The model under review builds one solid part; all positions refer to its coordinate system, in mm. Face numbers are marked on the shaded views. Coordinates: 2 decimals unless noted, no trailing zeros. Order: outer loops, then holes, each group sorted by start corner. A loop starts at its lowest first (then second) coordinate and runs counter-clockwise, first axis right, second up. Notation, with made-up numbers: (32, 23.25) -> (54, 23.25) arc R23 ccw to (54, 50.25) -> close; hole circle Ø5 at (53.25, -30). An arc over 180 degrees is marked (long way). Put each result on its own line as item: value.
from build123d import *

# Parameters (mm, degrees)
SKETCH1_R             = 100
SKETCH1_R_2           = 40
BOSS_EXTRUDE1_DEPTH   = 5
F_4_0MM_DOWEL_HOLE1_D = 4
SKETCH6_R             = 95
SKETCH6_R_2           = 90
BOSS_EXTRUDE2_DEPTH   = 10
F_4_0MM_DOWEL_HOLE2_D = 4
CUT_EXTRUDE1_DEPTH    = 142.774468788
CIRPATTERN1_DEPTH     = 5
CUT_EXTRUDE2_START    = -10
SKETCH10_R            = 95
SKETCH10_R_2          = 94.5
CUT_EXTRUDE2_DEPTH    = 10
BOSS_EXTRUDE3_DEPTH   = 10


# Read off the part's stored shape, not the designer's step: CirPattern1
with BuildPart() as part:
    # Sketch1 → Boss-Extrude1 (new body)
    with BuildSketch(Plane(origin=(0, 0, 0), x_dir=(1, 0, 0), z_dir=(0, 1, 0))):
        with Locations(Location((0, 0, 0), (0, 0, 270))):
            Circle(SKETCH1_R)
        with Locations(Location((0, 0, 0), (0, 0, 270))):
            Circle(SKETCH1_R_2, mode=Mode.SUBTRACT)
    extrude(amount=BOSS_EXTRUDE1_DEPTH)

    # Ø4.0mm Dowel Hole1 (through all)
    with Locations(Plane(origin=(0, 5, 0), x_dir=(1, 0, 0), z_dir=(0, 1, 0))):
        with Locations((0, 0), (40.5, 40.5), (-40.5, -40.5), (-40.5, 40.5), (40.5, -40.5)):
            Hole(F_4_0MM_DOWEL_HOLE1_D / 2)

    # Sketch6 → Boss-Extrude2 (add)
    with BuildSketch(Plane(origin=(0, 5, 0), x_dir=(1, 0, 0), z_dir=(0, 1, 0))):
        with Locations(Location((0, 0, 0), (0, 0, 270))):
            Circle(SKETCH6_R)
        with Locations(Location((0, 0, 0), (0, 0, 270))):
            Circle(SKETCH6_R_2, mode=Mode.SUBTRACT)
    extrude(amount=BOSS_EXTRUDE2_DEPTH)

    # Ø4.0mm Dowel Hole2 (through all)
    with Locations(Plane(origin=(0, 5, 0), x_dir=(1, 0, 0), z_dir=(0, 1, 0))):
        with Locations((0, 0), (75, 20), (-75, -20), (-75, 20), (75, -20), (20, 75), (-20, -75), (-20, 75), (20, -75), (20, 55), (-20, -55), (-20, 55), (20, -55), (55, -20), (-55, 20), (-55, -20), (55, 20)):
            Hole(F_4_0MM_DOWEL_HOLE2_D / 2)

    # Sketch9 → Cut-Extrude1 (cut, through all)
    with BuildSketch(Plane(origin=(0, 5, 0), x_dir=(1, 0, 0), z_dir=(0, 1, 0))):
        with BuildLine():
            Line((81.567700833, -38.035643557), (59.537983888, -27.763017838))
            ThreePointArc((59.537983888, -27.763017838), (46.451892776, -46.451892776), (27.763017838, -59.537983888))
            Line((27.763017838, -59.537983888), (38.035643557, -81.567700833))
            ThreePointArc((38.035643557, -81.567700833), (63.639610307, -63.639610307), (81.567700833, -38.035643557))
        make_face()
    extrude(amount=-CUT_EXTRUDE1_DEPTH, mode=Mode.SUBTRACT)

    # CirPattern1 outline → CirPattern1 (cut)
    with BuildSketch(Plane(origin=(0, 0, 0), x_dir=(1, 0, 0), z_dir=(0, 1, 0))):
        with BuildLine():
            Line((59.537983888, 27.763017838), (81.567700833, 38.035643557))
            ThreePointArc((81.567700833, 38.035643557), (63.639610307, 63.639610307), (38.035643557, 81.567700833))
            Line((38.035643557, 81.567700833), (27.763017838, 59.537983888))
            ThreePointArc((27.763017838, 59.537983888), (46.451892776, 46.451892776), (59.537983888, 27.763017838))
        make_face()
        with BuildLine():
            ThreePointArc((-81.567700833, -38.035643557), (-63.639610307, -63.639610307), (-38.035643557, -81.567700833))
            Line((-38.035643557, -81.567700833), (-27.763017838, -59.537983888))
            ThreePointArc((-27.763017838, -59.537983888), (-46.451892776, -46.451892776), (-59.537983888, -27.763017838))
            Line((-59.537983888, -27.763017838), (-81.567700833, -38.035643557))
        make_face()
        with BuildLine():
            Line((-27.763017838, 59.537983888), (-38.035643557, 81.567700833))
            ThreePointArc((-38.035643557, 81.567700833), (-63.639610307, 63.639610307), (-81.567700833, 38.035643557))
            Line((-81.567700833, 38.035643557), (-59.537983888, 27.763017838))
            ThreePointArc((-59.537983888, 27.763017838), (-46.451892776, 46.451892776), (-27.763017838, 59.537983888))
        make_face()
    extrude(amount=CIRPATTERN1_DEPTH, mode=Mode.SUBTRACT)

    # Sketch10 → Cut-Extrude2 (cut)
    with BuildSketch(Plane(origin=(0, 15, 0), x_dir=(1, 0, 0), z_dir=(0, 1, 0)).offset(CUT_EXTRUDE2_START)):
        Circle(SKETCH10_R)
        with Locations(Location((0, 0, 0), (0, 0, 270))):
            Circle(SKETCH10_R_2, mode=Mode.SUBTRACT)
    extrude(amount=CUT_EXTRUDE2_DEPTH, mode=Mode.SUBTRACT)

    # Sketch11 → Boss-Extrude3 (add)
    with BuildSketch(Plane(origin=(0, 5, 0), x_dir=(1, 0, 0), z_dir=(0, 1, 0))):
        with BuildLine():
            Line((93.301929241, -15), (96.33924434, -15))
            Line((96.33924434, -15), (96.33924434, 15))
            Line((96.33924434, 15), (93.301929241, 15))
            ThreePointArc((93.301929241, 15), (94.200006139, 7.52388486), (94.5, 0))
            ThreePointArc((94.5, 0), (94.200006139, -7.52388486), (93.301929241, -15))
        make_face()
        with BuildLine():
            Line((96.33924434, 15), (96.33924434, -15))
            ThreePointArc((96.33924434, -15), (97.209377951, -7.522422378), (97.5, 0))
            ThreePointArc((97.5, 0), (97.209377951, 7.522422378), (96.33924434, 15))
        make_face()
    extrude(amount=BOSS_EXTRUDE3_DEPTH)


solid = part.part
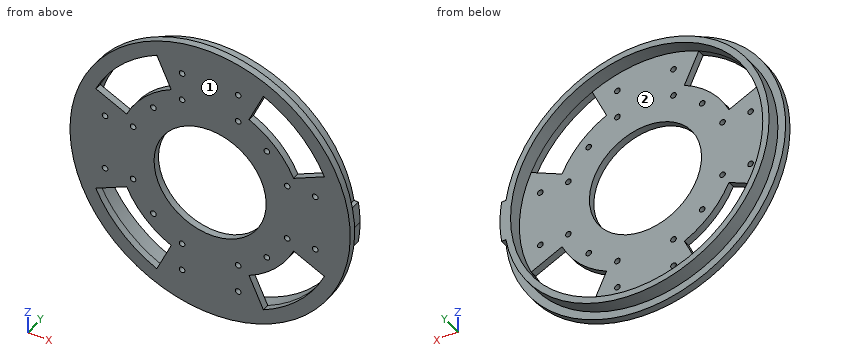
Item 1: For line 1 (Z direction, x = 0, y = 11); line 2 (Z direction, x = 64, y = 4.5); line 3 (X direction, y = 11.75, z = 0), list the stretches that pass through material, from the lowest coordinate up. Write a range as from..to.
Answers below:
line 1: -94.5..-90, 90..94.5
line 2: -76.84..-63.28, -29.84..29.84, 63.28..76.84
line 3: -94.5..-90, 90..97.5
Item 2: Consider section B-B on z = 64. Write out the cut boundary in (x, y), and give its area (3 significant figures).
Answers below:
outline: (-76.84, 0) -> (-63.28, 0) -> (-63.28, 15) -> (-69.53, 15) -> (-69.53, 5) -> (-76.84, 5) -> close; (-29.84, 0) -> (29.84, 0) -> (29.84, 5) -> (-29.84, 5) -> close; (63.28, 0) -> (76.84, 0) -> (76.84, 5) -> (69.53, 5) -> (69.53, 15) -> (63.28, 15) -> close
area: 559 mm^2
Item 3: Consider section A-A on y = 9. Write out the cut boundary in (x, z).
Answers below:
outline: (93.3, -15) -> (96.34, -15) arc R97.5 ccw to (96.34, 15) -> (93.3, 15) arc R94.5 ccw (long way) to start; hole circle Ø180 at (0, 0)
Item 4: For pin 1 Ø6 at (y, z) = (10, -29.5) entering from +X; pin 2 Ø2 at (y, z) = (7, -45) entering from -X; pin 3 Ø4.5 at (x, z) = (-20, -75) entering from +Y; pin 4 Ø2.5 at (x, z) = (20, 75) entering from -Y, all flat-tipped, find the tip position at first contact; note any pin that passes through.
Answers below:
pin 1: x = 90.71
pin 2: x = -83.63
pin 3: y = 5
pin 4: through
Item 5: Consider section C-C on x = -3. Write out the cut boundary in (y, z).
Answers below:
outline: (0, -99.95) -> (5, -99.95) -> (5, -94.45) -> (15, -94.45) -> (15, -89.95) -> (5, -89.95) -> (5, -39.89) -> (0, -39.89) -> close; (0, 39.89) -> (5, 39.89) -> (5, 89.95) -> (15, 89.95) -> (15, 94.45) -> (5, 94.45) -> (5, 99.95) -> (0, 99.95) -> close
Item 6: Consider section D-D on z = 12. Write out the cut boundary in (x, y) (3 decimals).
Answers below:
outline: (-99.277, 0) -> (-38.158, 0) -> (-38.158, 5) -> (-89.196, 5) -> (-89.196, 15) -> (-93.735, 15) -> (-93.735, 5) -> (-99.277, 5) -> close; (38.158, 0) -> (99.277, 0) -> (99.277, 5) -> (96.759, 5) -> (96.759, 15) -> (89.196, 15) -> (89.196, 5) -> (38.158, 5) -> close
Item 7: Mouldability with a two-part tool opening along Z and no side actions: class the marked faces 1 and 2 as +Z half, -Z half, draft (parallel to the pull), parting line (faces both ways), or undercut.
Answers below:
face 1: draft
face 2: undercut
